from build123d import *

# Parameters (mm, degrees)
ESQUISSE1_R        = 7.5
BOSS_EXTRU_1_DEPTH = 45
ESQUISSE2_R        = 11.5
BOSS_EXTRU_2_DEPTH = 3
BOSS_EXTRU_3_START = 45
ESQUISSE3_R        = 6.5
BOSS_EXTRU_3_DEPTH = 2
BOSS_EXTRU_4_START = 47
ESQUISSE4_R        = 7.5
BOSS_EXTRU_4_DEPTH = 3
CONG_1_R           = 1


with BuildPart() as part:
    # Esquisse1 → Boss.-Extru.1 (new body)
    with BuildSketch(Plane.XY):
        Circle(ESQUISSE1_R)
    extrude(amount=BOSS_EXTRU_1_DEPTH)

    # Esquisse2 → Boss.-Extru.2 (add)
    with BuildSketch(Plane.XY):
        Circle(ESQUISSE2_R)
    extrude(amount=BOSS_EXTRU_2_DEPTH)

    # Esquisse3 → Boss.-Extru.3 (add)
    with BuildSketch(Plane.XY.offset(BOSS_EXTRU_3_START)):
        Circle(ESQUISSE3_R)
    extrude(amount=BOSS_EXTRU_3_DEPTH)

    # Esquisse4 → Boss.-Extru.4 (add)
    with BuildSketch(Plane.XY.offset(BOSS_EXTRU_4_START)):
        Circle(ESQUISSE4_R)
    extrude(amount=BOSS_EXTRU_4_DEPTH)

    # Congé1
    cong_1_edges = [part.edges().sort_by_distance(p)[0] for p in [
        (-7.5, 0, 50),
    ]]
    fillet(cong_1_edges, radius=CONG_1_R)


solid = part.part
Source: CAD feature listing. Evaluate the final solid. Frame: model axes, mm. A direction names the side the tool comes from. Coordinates: 2 decimals unless noted, no trailing zeros. Loops run counter-clockwise (first coordinate to the right, second up) from the corner with the lowest first, then second, coordinate; pieces in that order, holes last. Notation, with made-up numbers: (30, 17) - (75, 17) arc R26 cw to (75, 38) - close; hole circle Ø3 at (87, 64). An arc over 180 degrees is marked (long way). One line per item, written item: value. Start each with the question number.
1. Section C-C (z = 7.5). Return the cut outline in (x, y).
2. Ray query, L1, parallel to Z at x = -8, y = 5.25; L2, parallel to Z at x = -6, y = 4; L3, parallel to Y at x = 0.25, z = 2. Return the intervals inside material, ascending.
3. Set-up query: faces 5 (the cylindrical face through (-1.5, 11.4, 1.5)), 6 (the flat face through (8, 0, 3)), 7 (the cylindrical face through (-5.158, -3.955, 45.986)). Return all of +Z, -Z, +X, -X, +Y, -Y with unobstructed straight access to the full face (end or side cutting, diameter ignored); none if empty.
4. Contact query for flat-ended pins moving along their axis: P1, Ø1.5, axis at x = 5, z = 14.5, coming from the +Y side; P2, Ø1.5, axis at x = -1.5, z = 17.5, coming from the -Y side; P3, Ø10, axis at y = -8, z = 26.5, coming from the -X side. Output: stop coordinate, or through.
5. Section A-A (x = 0). Return the cut outline in (y, z).
6. Mould query, pull axis Z, two halves, no side actions, for faces 1 (the flat face through (0, 0, 0)), 2 (the cylindrical face through (-7.493, 0.33, 47.986)), 3 (the flat face through (-6, 3, 45)), 4 (the flat face through (-6, 3, 47)). Classes: pulls with the +Z half, pulls with the -Z half, needs draft (parallel to the pull), parting line crosses it, or undercut.
Verdict:
1. outline: circle Ø15 at (0, 0)
2. L1: z = 0 to 3
2. L2: z = 0 to 45, 47 to 49.7
2. L3: y = -11.5 to 11.5
3. face 5: +Z, -Z
3. face 6: +Z
3. face 7: none
4. P1: stops at y = 6.18
4. P2: stops at y = -7.46
4. P3: stops at x = -6.87
5. outline: (-11.5, 0) - (11.5, 0) - (11.5, 3) - (7.5, 3) - (7.5, 45) - (6.5, 45) - (6.5, 47) - (7.5, 47) - (7.5, 49) arc R1 ccw to (6.5, 50) - (-6.5, 50) arc R1 ccw to (-7.5, 49) - (-7.5, 47) - (-6.5, 47) - (-6.5, 45) - (-7.5, 45) - (-7.5, 3) - (-11.5, 3) - close
6. face 1: pulls with the -Z half
6. face 2: needs draft
6. face 3: undercut
6. face 4: undercut
